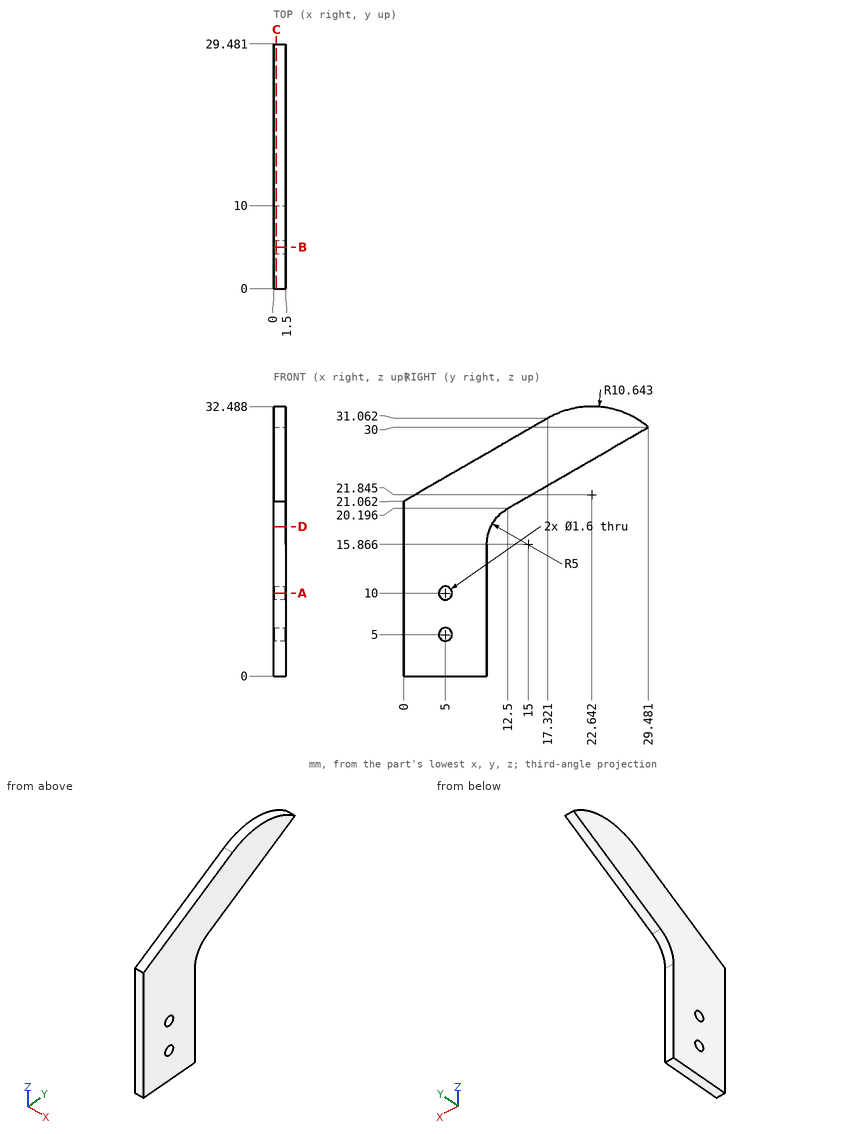
Input: dimensioned drawing with shaded views. Units: mm. Origin: part minimum x, y, z. Round coordinates to 2 decimals unless told otherwise and drop trailing zeros. Loops run counter-clockwise (first coordinate to the right, second up) from the corner with the lowest first, then second, coordinate; pieces in that order, holes last. Notation, with made-up numbers: (-6, 68.25) -> (31, 68.25) arc R22 cw to (31, 93.25) -> close; hole circle Ø1 at (19, -5.5). An arc over 180 degrees is marked (long way). Answer as a JSON object with one key per item and string values. Group by question number.
1) Section query D-D on z = 18. Output: boundary loops of the cut face in (x, y), plus the area to 3 significant figures.
2) Section query B-B on y = 5. Output: boundary loops of the cut face in (x, z).
3) Section query C-C on x = 0.35. Output: boundary loops of the cut face in (y, z) (1 decimal), plus the area to 3 significant figures.
4) Section query A-A on z = 10. Output: boundary loops of the cut face in (x, y), plus the area to 3 significant figures.
5) Ray query, L1, parallel to Y at x = 0.5, z = 5; L2, parallel to Y at x = 1.15, z = 14; L3, parallel to Z at x = 1, y = 10.75 (1 decimal). Return the intervals inside material, ascending.
Reply:
{
 "1": {"outline": "(0, 0) -> (1.5, 0) -> (1.5, 10.48) -> (0, 10.48) -> close", "area": "15.7 mm2"},
 "2": {"outline": "(0, 0) -> (1.5, 0) -> (1.5, 4.2) -> (0, 4.2) -> close; (0, 5.8) -> (1.5, 5.8) -> (1.5, 9.2) -> (0, 9.2) -> close; (0, 10.8) -> (1.5, 10.8) -> (1.5, 23.95) -> (0, 23.95) -> close"},
 "3": {"outline": "(0, 0) -> (10, 0) -> (10, 15.9) arc R5 cw to (12.5, 20.2) -> (29.5, 30) arc R10.6 ccw to (17.3, 31.1) -> (0, 21.1) -> close; hole circle Ø1.6 at (5, 5); hole circle Ø1.6 at (5, 10)", "area": "361 mm2"},
 "4": {"outline": "(0, 0) -> (1.5, 0) -> (1.5, 4.2) -> (0, 4.2) -> close; (0, 5.8) -> (1.5, 5.8) -> (1.5, 10) -> (0, 10) -> close", "area": "12.6 mm2"},
 "5": {"L1": "y = 0 to 4.2, 5.8 to 10", "L2": "y = 0 to 10", "L3": "z = 18.5 to 27.3"}
}
